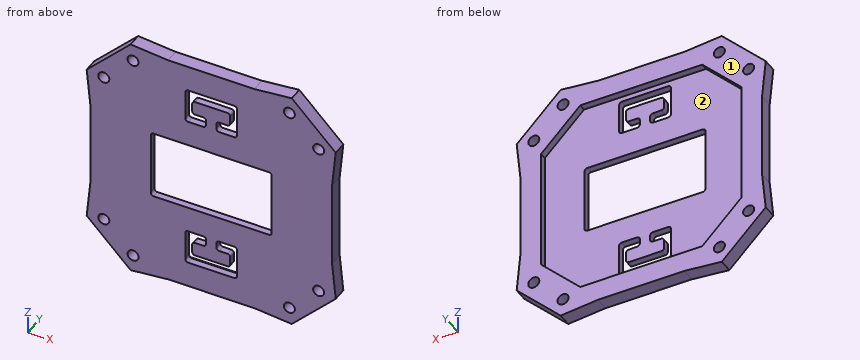
from build123d import *

# Parameters (mm, degrees)
BOSS_EXTRUDE1_DEPTH = 4
SKETCH2_R           = 1.6
CUT_EXTRUDE1_DEPTH  = 5
CUT_EXTRUDE2_DEPTH  = 2
CUT_EXTRUDE3_DEPTH  = 3


with BuildPart() as part:
    # Sketch1 → Boss-Extrude1 (new body)
    with BuildSketch(Plane(origin=(0, 0, 0), x_dir=(1, 0, 0), z_dir=(0, 1, 0))):
        Polygon((-12.5, 0), (12.5, 0), (23.338026386, 1.062677778), (36.065948447, -11.665244283), (35.003270669, -22.503270669), (35.003270669, -47.503270669), (36.065948447, -58.341297055), (23.338026386, -71.069219116), (12.5, -70.006541338), (-12.5, -70.006541338), (-23.338026386, -71.069219116), (-36.065948447, -58.341297055), (-35.003270669, -47.503270669), (-35.003270669, -22.503270669), (-36.065948447, -11.665244283), (-23.338026386, 1.062677778), align=None)
    extrude(amount=BOSS_EXTRUDE1_DEPTH)

    # Sketch2 → Cut-Extrude1 (cut, through all)
    with BuildSketch(Plane(origin=(0, 4, 0), x_dir=(1, 0, 0), z_dir=(0, 1, 0))):
        with Locations((22.63, -3.893270669)):
            Circle(SKETCH2_R)
        with Locations((31.11, -12.373270669)):
            Circle(SKETCH2_R)
        with Locations((-31.11, -12.373270669)):
            Circle(SKETCH2_R)
        with Locations((-22.63, -3.893270669)):
            Circle(SKETCH2_R)
        with Locations((31.11, -57.633270669)):
            Circle(SKETCH2_R)
        with Locations((22.63, -66.113270669)):
            Circle(SKETCH2_R)
        with Locations((-22.63, -66.113270669)):
            Circle(SKETCH2_R)
        with Locations((-31.11, -57.633270669)):
            Circle(SKETCH2_R)
    extrude(amount=-CUT_EXTRUDE1_DEPTH, mode=Mode.SUBTRACT)

    # Sketch3 → Cut-Extrude2 (cut)
    with BuildSketch(Plane(origin=(0, 4, 0), x_dir=(1, 0, 0), z_dir=(0, 1, 0))):
        Polygon((-17.672782103, -6), (17.672782103, -6), (29.003270669, -17.330488566), (29.003270669, -52.676052772), (17.672782103, -64.006541338), (-17.672782103, -64.006541338), (-29.003270669, -52.676052772), (-29.003270669, -17.330488566), align=None)
    extrude(amount=-CUT_EXTRUDE2_DEPTH, mode=Mode.SUBTRACT)

    # Sketch4 → Cut-Extrude3 (cut, through all)
    with BuildSketch(Plane(origin=(0, 2, 0), x_dir=(1, 0, 0), z_dir=(0, 1, 0))):
        with BuildLine():
            Line((-16.7, -45.003270669), (16.7, -45.003270669))
            ThreePointArc((16.7, -45.003270669), (17.265685425, -44.768956094), (17.5, -44.203270669))
            Line((17.5, -44.203270669), (17.5, -25.803270669))
            ThreePointArc((17.5, -25.803270669), (17.265685425, -25.237585244), (16.7, -25.003270669))
            Line((16.7, -25.003270669), (-16.7, -25.003270669))
            ThreePointArc((-16.7, -25.003270669), (-17.265685425, -25.237585244), (-17.5, -25.803270669))
            Line((-17.5, -25.803270669), (-17.5, -44.203270669))
            ThreePointArc((-17.5, -44.203270669), (-17.265685425, -44.768956094), (-16.7, -45.003270669))
        make_face()
        with BuildLine():
            Line((-1.5, -16.703270669), (-1.5, -15.303270669))
            ThreePointArc((-1.5, -15.303270669), (-1.734314575, -14.737585244), (-2.3, -14.503270669))
            Line((-2.3, -14.503270669), (-4.7, -14.503270669))
            ThreePointArc((-4.7, -14.503270669), (-5.265685425, -14.268956094), (-5.5, -13.703270669))
            Line((-5.5, -13.703270669), (-5.5, -11.303270669))
            ThreePointArc((-5.5, -11.303270669), (-5.265685425, -10.737585244), (-4.7, -10.503270669))
            Line((-4.7, -10.503270669), (4.7, -10.503270669))
            ThreePointArc((4.7, -10.503270669), (5.265685425, -10.737585244), (5.5, -11.303270669))
            Line((5.5, -11.303270669), (5.5, -13.703270669))
            ThreePointArc((5.5, -13.703270669), (5.265685425, -14.268956094), (4.7, -14.503270669))
            Line((4.7, -14.503270669), (2.3, -14.503270669))
            ThreePointArc((2.3, -14.503270669), (1.734314575, -14.737585244), (1.5, -15.303270669))
            Line((1.5, -15.303270669), (1.5, -16.703270669))
            ThreePointArc((1.5, -16.703270669), (1.734314575, -17.268956094), (2.3, -17.503270669))
            Line((2.3, -17.503270669), (6.7, -17.503270669))
            ThreePointArc((6.7, -17.503270669), (7.265685425, -17.268956094), (7.5, -16.703270669))
            Line((7.5, -16.703270669), (7.5, -8.303270669))
            ThreePointArc((7.5, -8.303270669), (7.265685425, -7.737585244), (6.7, -7.503270669))
            Line((6.7, -7.503270669), (-6.7, -7.503270669))
            ThreePointArc((-6.7, -7.503270669), (-7.265685425, -7.737585244), (-7.5, -8.303270669))
            Line((-7.5, -8.303270669), (-7.5, -16.703270669))
            ThreePointArc((-7.5, -16.703270669), (-7.265685425, -17.268956094), (-6.7, -17.503270669))
            Line((-6.7, -17.503270669), (-2.3, -17.503270669))
            ThreePointArc((-2.3, -17.503270669), (-1.734314575, -17.268956094), (-1.5, -16.703270669))
        make_face()
        with BuildLine():
            Line((-5.5, -56.303270669), (-5.5, -58.703270669))
            ThreePointArc((-5.5, -58.703270669), (-5.265685425, -59.268956094), (-4.7, -59.503270669))
            Line((-4.7, -59.503270669), (4.7, -59.503270669))
            ThreePointArc((4.7, -59.503270669), (5.265685425, -59.268956094), (5.5, -58.703270669))
            Line((5.5, -58.703270669), (5.5, -56.303270669))
            ThreePointArc((5.5, -56.303270669), (5.265685425, -55.737585244), (4.7, -55.503270669))
            Line((4.7, -55.503270669), (2.3, -55.503270669))
            ThreePointArc((2.3, -55.503270669), (1.734314575, -55.268956094), (1.5, -54.703270669))
            Line((1.5, -54.703270669), (1.5, -53.303270669))
            ThreePointArc((1.5, -53.303270669), (1.734314575, -52.737585244), (2.3, -52.503270669))
            Line((2.3, -52.503270669), (6.7, -52.503270669))
            ThreePointArc((6.7, -52.503270669), (7.265685425, -52.737585244), (7.5, -53.303270669))
            Line((7.5, -53.303270669), (7.5, -61.703270669))
            ThreePointArc((7.5, -61.703270669), (7.265685425, -62.268956094), (6.7, -62.503270669))
            Line((6.7, -62.503270669), (-6.7, -62.503270669))
            ThreePointArc((-6.7, -62.503270669), (-7.265685425, -62.268956094), (-7.5, -61.703270669))
            Line((-7.5, -61.703270669), (-7.5, -53.303270669))
            ThreePointArc((-7.5, -53.303270669), (-7.265685425, -52.737585244), (-6.7, -52.503270669))
            Line((-6.7, -52.503270669), (-2.3, -52.503270669))
            ThreePointArc((-2.3, -52.503270669), (-1.734314575, -52.737585244), (-1.5, -53.303270669))
            Line((-1.5, -53.303270669), (-1.5, -54.703270669))
            ThreePointArc((-1.5, -54.703270669), (-1.734314575, -55.268956094), (-2.3, -55.503270669))
            Line((-2.3, -55.503270669), (-4.7, -55.503270669))
            ThreePointArc((-4.7, -55.503270669), (-5.265685425, -55.737585244), (-5.5, -56.303270669))
        make_face()
    extrude(amount=-CUT_EXTRUDE3_DEPTH, mode=Mode.SUBTRACT)


solid = part.part
Build history of the part. All positions in model axes, mm. Face numbers are marked on the shaded views. Give positions to 0.01 mm unless a question says otherwise; leave off trailing zeros. Loops run counter-clockwise (first coordinate to the right, second up) from the corner with the lowest first, then second, coordinate; pieces in that order, holes last. Notation, with made-up numbers: (29, 22.5) -> (46, 22.5) arc R20 cw to (46, 46.5) -> close; hole circle Ø1 at (44.5, 89.5). An arc over 180 degrees is marked (long way). Answer in a Markdown table with one row per item.
Item 1: Slice it at D-D on x = -31.11. Write the cut outline in (y, z).
Findings below:
| item | result |
|---|---|
| outline | (0, 6.71) -> (4, 6.71) -> (4, 10.77) -> (0, 10.77) -> close; (0, 13.97) -> (4, 13.97) -> (4, 56.03) -> (0, 56.03) -> close; (0, 59.23) -> (4, 59.23) -> (4, 63.3) -> (0, 63.3) -> close |
Item 2: Probe line 1 along X through (y, z) = (1.7, 16.5); line 2 along Z through (x, y) = (-31.11, 3.05); line 3 along Z through (x, y) = (22.63, 1.95). List the from-to ranges inside material, lowest first. Write a range as [from, to].
Findings below:
| item | result |
|---|---|
| line 1 | x = [-35.59, -7.5], [-1.5, 1.5], [7.5, 35.59] |
| line 2 | z = [6.71, 10.77], [13.97, 56.03], [59.23, 63.3] |
| line 3 | z = [-0.99, 2.29], [5.49, 64.51], [67.71, 71] |
Item 3: Slice it at B-B on z = 40.5. Write the cut outline in (x, y), plus the area to 3 significant figures.
Findings below:
| item | result |
|---|---|
| outline | (-35, 0) -> (-17.5, 0) -> (-17.5, 2) -> (-29, 2) -> (-29, 4) -> (-35, 4) -> close; (17.5, 0) -> (35, 0) -> (35, 4) -> (29, 4) -> (29, 2) -> (17.5, 2) -> close |
| area | 94.0 mm² |
Item 4: Flat gauge pins, fed straight in: P1, Ø2, axis at x = 7, y = 3.5, coming from the -Z side; P2, Ø6, axis at x = 16, z = 12.5, coming from the +Y side; P3, Ø1, axis at y = 1.5, z = 33.5, coming from the -X side; P4, Ø6, axis at x = 10.5, z = 29.5, coming from the +Y side. Where does each tip first touch, or does it go through?
Findings below:
| item | result |
|---|---|
| P1 | stops at z = 0 |
| P2 | stops at y = 2 |
| P3 | stops at x = -35 |
| P4 | passes through |
Item 5: Slice it at A-A on x = 0.5. Write the cut outline in (y, z).
Findings below:
| item | result |
|---|---|
| outline | (0, 0) -> (4, 0) -> (4, 6) -> (2, 6) -> (2, 7.5) -> (0, 7.5) -> close; (0, 10.5) -> (2, 10.5) -> (2, 25) -> (0, 25) -> close; (0, 45) -> (2, 45) -> (2, 59.5) -> (0, 59.5) -> close; (0, 62.5) -> (2, 62.5) -> (2, 64.01) -> (4, 64.01) -> (4, 70.01) -> (0, 70.01) -> close |
Item 6: Mould opens along Z. For the marked faces 1 and 2 say: pulls with the +Z half, pulls with the -Z half, needs draft (parallel to the pull), parting line crosses it, or undercut.
Findings below:
| item | result |
|---|---|
| face 1 | needs draft |
| face 2 | undercut |
Item 7: Slice it at C-C on x = 22.5. Write the cut outline in (y, z).
Findings below:
| item | result |
|---|---|
| outline | (0, -0.98) -> (4, -0.98) -> (4, 2.3) -> (0, 2.3) -> close; (0, 5.49) -> (4, 5.49) -> (4, 10.83) -> (2, 10.83) -> (2, 59.18) -> (4, 59.18) -> (4, 64.52) -> (0, 64.52) -> close; (0, 67.71) -> (4, 67.71) -> (4, 70.99) -> (0, 70.99) -> close |
